The figure shows three views and two pictorial views of one solid part (mm, origin at its lowest corner). Answer the questions. Round coordinates to 2 decimals unless told otherwise and drop trailing zeros. Loops run counter-clockwise (first coordinate to the right, second up) from the corner with the lowest first, then second, coordinate; pieces in that order, holes last. Notation, with made-up numbers: (57, 60.25) -> (70, 60.25) arc R21 cw to (70, 82.25) -> close; hole circle Ø11 at (-32.5, -15). An arc over 180 degrees is marked (long way). Use a Markdown table: item, result. Add a question column.
Q1. Section A-A on z = 100 is taken. Give the vertices of the cut face in (x, y), then the cut area to 3 significant figures.
Q2. Consider line 1 (Z direction, x = 9.6, y = 5); line 2 (Y direction, x = 8.25, z = 23.5). Determine where each line is inside the solid, lowest interval first.
Q3. Section B-B on x = 7.75 is taken. Give the vertices of the cut face in (y, z), then the cut area to 3 significant figures.
Q4. Given pin 1 Ø3.5 at (y, z) = (5, 100) entering from +X, flat-ended and moving along its own axis, determine where the tip first touches the part or whether it passes through.
Q5. Section C-C on y = 5 is taken. Give the number of separate pieces and of enclosed holes in the cut face, then the cut area to 3 significant figures.
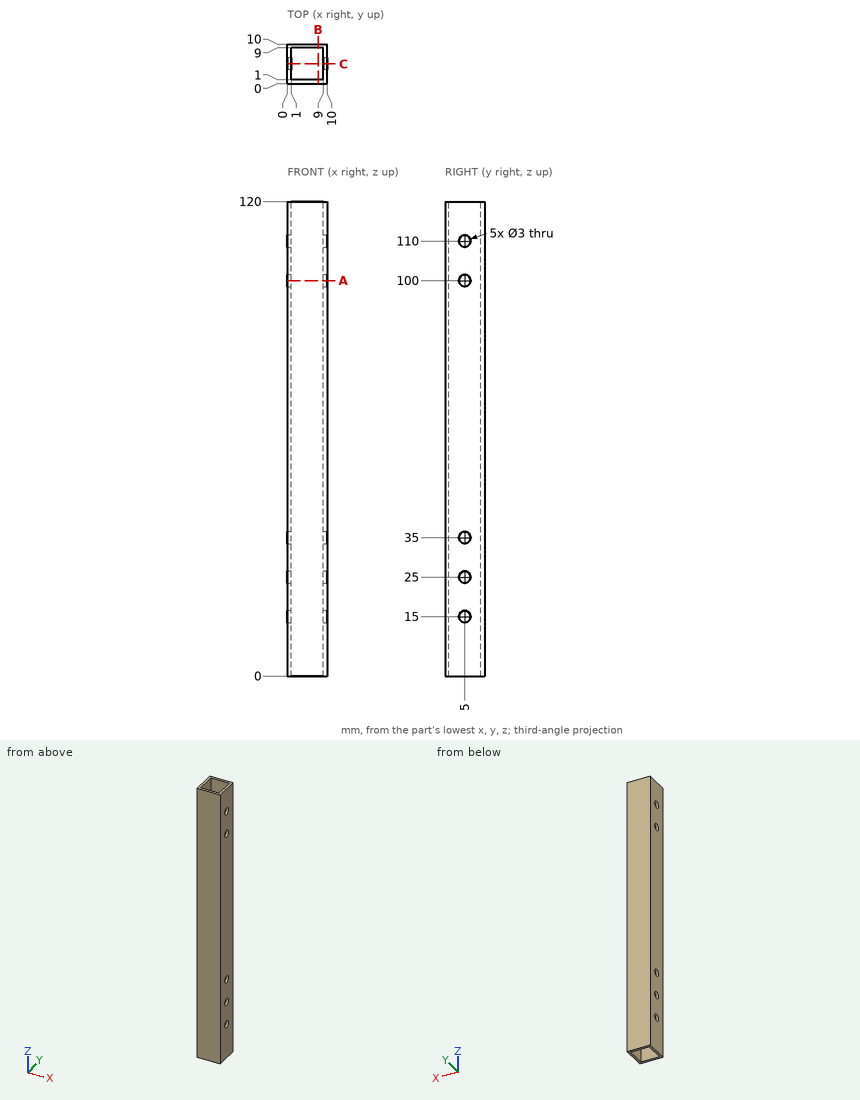
Checked values:
| question | item | result |
|---|---|---|
| 1 | outline | (0, 0) -> (10, 0) -> (10, 3.5) -> (9, 3.5) -> (9, 1) -> (1, 1) -> (1, 3.5) -> (0, 3.5) -> close; (0, 6.5) -> (1, 6.5) -> (1, 9) -> (9, 9) -> (9, 6.5) -> (10, 6.5) -> (10, 10) -> (0, 10) -> close |
| 1 | area | 30.0 mm2 |
| 2 | line 1 | z = 0 to 13.5, 16.5 to 23.5, 26.5 to 33.5, 36.5 to 98.5, 101.5 to 108.5, 111.5 to 120 |
| 2 | line 2 | y = 0 to 1, 9 to 10 |
| 3 | outline | (0, 0) -> (1, 0) -> (1, 120) -> (0, 120) -> close; (9, 0) -> (10, 0) -> (10, 120) -> (9, 120) -> close |
| 3 | area | 240 mm2 |
| 4 | pin 1 | stops at x = 10 |
| 5 | separate pieces | 12 |
| 5 | enclosed holes | 0 |
| 5 | area | 210 mm2 |
